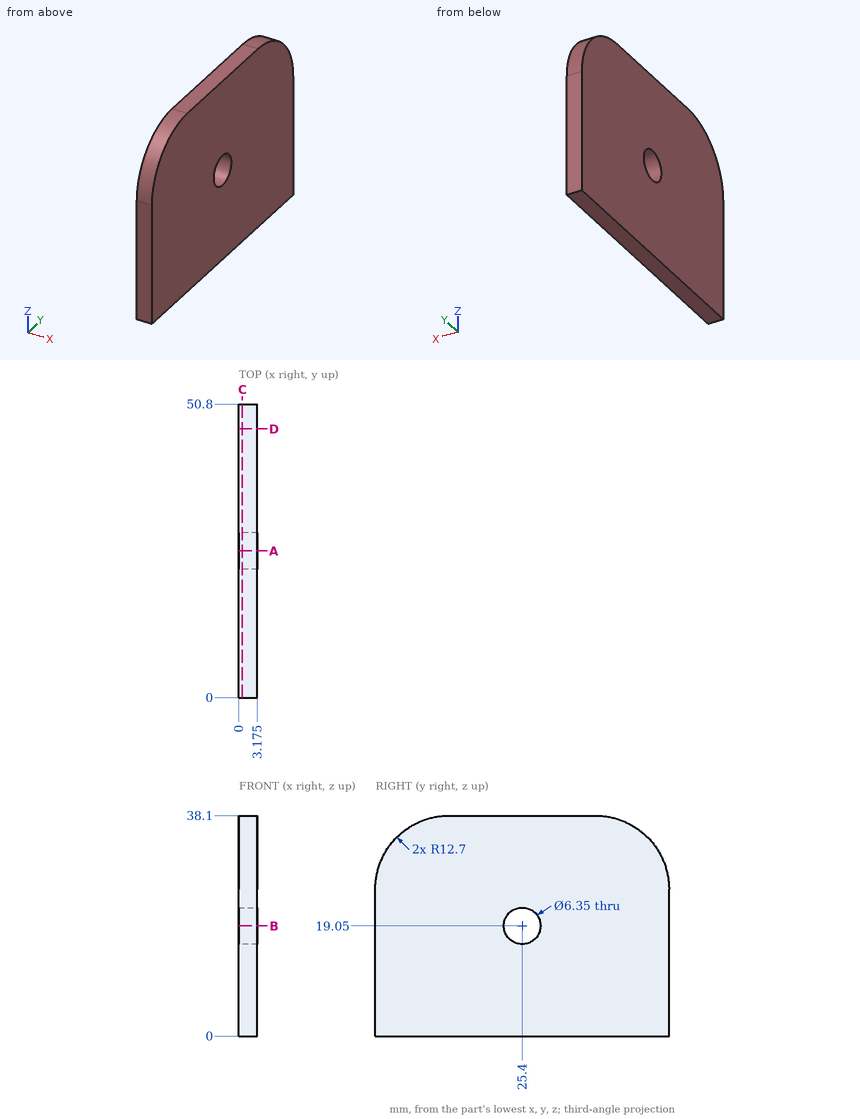
Part print with two shaded views. Sizes in mm from the minimum x, y, z corner. Round coordinates to 2 decimals unless told otherwise and drop trailing zeros. Write each loop counter-clockwise with the first axis right and the second up, starting at its lowest first coordinate (ties: lowest second). Pieces come first, ordered by that corner, then holes. Notation, with made-up numbers: (32, 66) - (88, 66) arc R21 ccw to (88, 81) - close; hole circle Ø9 at (6.5, 46). An arc over 180 degrees is marked (long way). Use CSV: the item, a comma, the result in double quotes.
Item 1: Flat gauge pin, fed straight in: P1, Ø5.5, axis at y = 25.4, z = 19.05, coming from the +X side. Where does the tip first touch, or does it go through?
Results list:
P1,"passes through"
Item 2: Slice it at C-C, the plane x = 0.6. Write the cut outline in (y, z) (3 decimals).
Results list:
outline,"(0, 0) - (50.8, 0) - (50.8, 25.4) arc R12.7 ccw to (38.1, 38.1) - (12.7, 38.1) arc R12.7 ccw to (0, 25.4) - close; hole circle Ø6.35 at (25.4, 19.05)"
Item 3: Slice it at B-B, the plane z = 19.05. Write the cut outline in (x, y) (3 decimals), then the cut area to 3 significant figures.
Results list:
outline,"(0, 0) - (3.175, 0) - (3.175, 22.225) - (0, 22.225) - close; (0, 28.575) - (3.175, 28.575) - (3.175, 50.8) - (0, 50.8) - close"
area,"141 mm²"
Item 4: Slice it at A-A, the plane y = 25.4. Write the cut outline in (x, z) (3 decimals), then the cut area to 3 significant figures.
Results list:
outline,"(0, 0) - (3.175, 0) - (3.175, 15.875) - (0, 15.875) - close; (0, 22.225) - (3.175, 22.225) - (3.175, 38.1) - (0, 38.1) - close"
area,"101 mm²"
Item 5: Wall check: L1, parallel to Y at x = 1, z = 19.05 (3 decimals); L2, parallel to Z at x = 1.65, y = 10.5; L3, parallel to Z at x = 2.3, y = 46. Give the ranges that are in metal, low to high.
Results list:
L1,"y = 0 to 22.225, 28.575 to 50.8"
L2,"z = 0 to 37.91"
L3,"z = 0 to 35.34"
Item 6: Slice it at D-D, the plane y = 46.5. Write the cut outline in (x, z) (3 decimals), then the cut area to 3 significant figures.
Results list:
outline,"(0, 0) - (3.175, 0) - (3.175, 34.925) - (0, 34.925) - close"
area,"111 mm²"
